Autodesk Inventor part; units mm, degrees
ref_plane "Work Plane1" through (0, 0, 0) normal (0, 0, 1) x (1, 0, 0)
ref_plane "YZ Plane" through (0, 0, 0) normal (1, 0, 0) x (0, 1, 0)
ref_plane "XZ Plane" through (0, 0, 0) normal (0, 1, 0) x (-1, 0, 0)
ref_plane "Work Plane1" through (0, 0, 0) normal (0, 0, 1) x (1, 0, 0)
sketch "Sketch1" plane through (0, 0, 0) normal (0, 0, 1) x (1, 0, 0)
  line L0 (0, 14.859) -> (-322.453, 14.859) construction
  line L1 (-0.635, 0) -> (-321.818, 0) construction
  line L2 (0, 14.859) -> (0, 0.635) construction
  line L3 (2.54, 14.859) -> (2.54, 0) construction
  line L4 (2.54, 14.859) -> (17.399, 14.859) construction
  line L5 (2.54, 0) -> (-51.4985, 0)
  line L6 (13.7371, 14.859) -> (-30.6705, 14.859) construction
  circle A0 centre (-4.7625, 4.7625) radius 1.778 construction
  line L7 (-7.62, 0) -> (-7.62, 14.859) construction
  circle A1 centre (-24.3205, 4.7625) radius 1.778 construction
  circle A2 centre (-43.8785, 4.7625) radius 1.778 construction
  circle A3 centre (-24.3205, 4.7625) radius 1.9685
  circle A4 centre (-43.8785, 4.7625) radius 1.9685
  line L8 (-51.4985, 0) -> (-51.4985, 14.859)
  circle A5 centre (-24.3205, 4.7625) radius 4.8768 construction
  circle A6 centre (-43.8785, 4.7625) radius 4.8768 construction
  line L9 (13.7371, 14.859) -> (-51.4985, 14.859)
  line L10 (2.54, 0) -> (13.7371, 14.859)
  line L11 (2.54, 0) -> (21.1455, 0) construction
  point P0 (0, 0)
  dimension "d1" = 2.54
  dimension "d7" = 10.16
  dimension "d9" = 3.937
  dimension "d10" = 3.937
  dimension "d11" = 7.62
  dimension "d12" = 9.7536
  dimension "d13" = 9.7536
  dimension "d46" = 53
extrude "Extrusion1" add sketch "Sketch1" along normal blind 10.16
sketch "Sketch2" plane through (0, 0, 10.16) normal (0, 0, 1) x (1, 0, 0)
  circle A0 centre (-24.3205, 4.7625) radius 1.9685 construction
  circle A1 centre (-43.8785, 4.7625) radius 1.9685 construction
  line L0 (13.7371, 14.859) -> (-51.4985, 14.859)
  line L1 (2.54, 0) -> (-7.62, 0)
  line L2 (3.5771, 14.859) -> (13.7371, 14.859)
  line L3 (2.54, 0) -> (13.7371, 14.859)
  line L4 (2.54, 0) -> (24.4372, 0) construction
  line L5 (-7.62, 0) -> (3.5771, 14.859)
  line L6 (-7.62, 0) -> (10.9855, 0) construction
  point P0 (0, 0)
  point P1 (2.54, 14.859)
  dimension "d35" = 53
  dimension "d45" = 53
extrude "Extrusion2" add sketch "Sketch2" along normal blind 63.5 and the other way blind 10.16
sketch "Sketch4" plane through (0, 0, 10.16) normal (0, 0, 1) x (1, 0, 0)
  circle A0 centre (-24.3205, 4.7625) radius 1.9685 construction
  circle A1 centre (-24.3205, 4.7625) radius 4.8768 construction
  point P0 (0, 0)
  dimension "d25" = 9.7536
sketch "Sketch7" plane through (13.7371, 14.859, 73.66) normal (0.7986, -0.6018, 0) x (0, 0, -1)
  line L0 (0, -18.6055) -> (0, 0) construction
  line L1 (0, -13.5255) -> (73.66, -13.5255) construction
  line L2 (73.66, -39.2597) -> (73.66, 0) construction
  line L3 (73.66, -18.6055) -> (0, -18.6055) construction
  circle A0 centre (10.16, -13.5255) radius 1.9685
  line L4 (73.66, -18.6055) -> (73.66, -51.1267)
  circle A1 centre (46.99, -13.5255) radius 1.9685
  point P0 (73.66, -20.1341)
  dimension "d38" = 5.08
  dimension "d39" = 3.937
  dimension "d40" = 63.5
  dimension "d41" = 3.937
  dimension "d42" = 26.67
extrude "Extrusion5" cut sketch "Sketch7" against normal through all
properties part number "Delivery bin right angle connector"
Work out the finished part from the listing and answer in its coordinate system (mm). A direction names the side the tool comes from. Round coordinates to 2 decimals unless told otherwise and drop trailing zeros. Write each loop counter-clockwise with the first axis right and the second up, starting at its lowest first coordinate (ties: lowest second). Pieces come first, ordered by that corner, then holes. Notation, with made-up numbers: (-13.5, 5.25) - (-7.5, 5.25) arc R7 cw to (-7.5, 17.25) - close; hole circle Ø5 at (46, 31). An arc over 180 degrees is marked (long way). Answer in a Markdown table with one row per item. Add a question column.
1. Find the intervals of material crossed by line 1 along Z through (x, y) = (-40, 11.5); line 2 along Y through (x, z) = (2, 62.5); line 3 along Y through (x, z) = (-2.5, 67), in increasing order. Write a range as from..to.
2. The mould has two halves that part along Z. Classify faces 1 (the cylindrical face through (1.95, 5.86, 24.85)), 2 (the flat face through (-19, 8, 0)), 3 (the flat face through (8.06, 7.325, 36.314)): +Z half, -Z half, draft (parallel to the pull), parting line (faces both ways), or undercut.
3. A cutting plane is placed at D-D, the plane x = -6.5. Determine the outline of the cut face in (y, z).
4. A cutting plane is placed at A-A, the plane x = -23.5. Determine the outline of the cut face in (y, z).
5. A cutting plane is placed at C-C, the plane z = 11.5. Determine the outline of the cut face in (x, y), and give its area (3 significant figures).
6. Given pin 1 (3 mm diameter, centred on x = -32, y = 9.5, fed in from +Z); pin 2 (4 mm diameter, centred on y = 12.5, z = 35, fed in from -X); pin 3 (6 mm diameter, centred on y = 7.5, z = 24.5, fed in from -X), each flat-ended and moving along its own axis, determine where each tip first touches the part or whether it passes through.
7. A cutting plane is placed at B-B, the plane z = 64. Determine the outline of the cut face in (x, y).
8. For faces 4 (the flat face through (-24, 8, 10.16)), 5 (the cylindrical face through (-22.443, 4.171, 5.009)), determine the directions among +Z, -Z, +X, -X, +Y, -Y from which every point of the face is accessible in a straight line to the end or side of a thin tool.
Worked out:
| question | item | result |
|---|---|---|
| 1 | line 1 | 0..10.16 |
| 1 | line 2 | 0..4.64, 8.89..12.77 |
| 1 | line 3 | 0..6.79 |
| 2 | face 1 | undercut |
| 2 | face 2 | -Z half |
| 2 | face 3 | draft |
| 3 | outline | (0, 0) - (14.86, 0) - (14.86, 10.16) - (1.49, 10.16) - (1.49, 73.66) - (0, 73.66) - close |
| 4 | outline | (0, 0) - (2.97, 0) - (2.97, 10.16) - (0, 10.16) - close; (6.55, 0) - (14.86, 0) - (14.86, 10.16) - (6.55, 10.16) - close |
| 5 | outline | (-7.62, 0) - (2.54, 0) - (13.74, 14.86) - (3.58, 14.86) - close |
| 5 | area | 151 mm^2 |
| 6 | pin 1 | z = 10.16 |
| 6 | pin 2 | x = 0.29 |
| 6 | pin 3 | x = -4.23 |
| 7 | outline | (-7.62, 0) - (2.54, 0) - (4.45, 2.54) - (-2.03, 7.42) - close; (0.26, 10.46) - (6.74, 5.58) - (13.74, 14.86) - (3.58, 14.86) - close |
| 8 | face 4 | +Z, -X, +Y |
| 8 | face 5 | +Z, -Z |
